```python
from build123d import *

# Parameters (mm, degrees)
F1_DEPTH = 47.752
F2_W     = 87.7630114555
F2_H     = 47.5155450404
F3_DEPTH = 32.004


with BuildPart() as f1:
    # F0 (on Right) → F1 (new body, symmetric)
    with BuildSketch(Plane.YZ):
        Polygon((-31.8501219153, 36.2352915108), (-27.2341612726, -24.6953871101), (43.6497934896, -30.3766369124), (46.6212034225, -24.6953871101), (-19.860636737, -19.3669606344), (-24.1173089374, 36.8211106937), align=None)
    extrude(amount=F1_DEPTH, both=True)

    # F2 (on face) → F3 (cut)
    with BuildSketch(Plane(origin=(0, -21.2061243549, -1.6065246214), x_dir=(-1, 0, 0), z_dir=(0, 0.9971426879, 0.075541115))):
        with Locations((0.0438690186, 10.5752218515)):
            Rectangle(F2_W, F2_H)
    extrude(amount=-F3_DEPTH, mode=Mode.SUBTRACT)


solid = f1.part
```
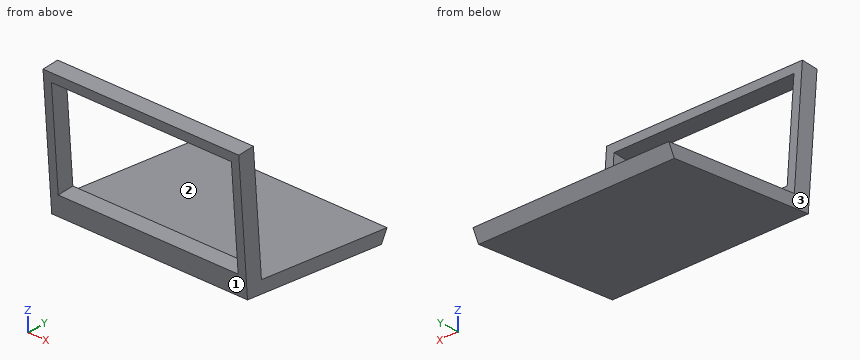
Work out the finished part from the listing and answer in its coordinate system (mm). Face numbers are marked on the shaded views. Round coordinates to 2 decimals unless told otherwise and drop trailing zeros. Order: outer loops, then holes, each group sorted by start corner. A loop starts at its lowest first (then second) coordinate and runs counter-clockwise, first axis right, second up.
Q1. The mould has two halves that part along Z. Classify the marked faces 1, 2 and 3: pulls with the +Z half, pulls with the -Z half, needs draft (parallel to the pull), parting line crosses it, or undercut.
Solution:
face 1: pulls with the -Z half
face 2: pulls with the +Z half
face 3: needs draft
Q2. A cutting plane is placed at A-A, the plane x = -36.5. Determine the outline of the cut face in (y, z), then the cut area to 3 significant figures.
Solution:
outline: (-31.85, 36.24) - (-31.53, 32.04) - (-23.8, 32.63) - (-24.12, 36.82) - close; (-27.94, -15.34) - (-27.23, -24.7) - (43.65, -30.38) - (46.62, -24.7) - (-19.86, -19.37) - (-20.21, -14.75) - close
area: 494 mm2
Q3. A cutting plane is placed at B-B, the plane z = 2. Determine the outline of the cut face in (x, y).
Solution:
outline: (-47.75, -29.26) - (-43.93, -29.26) - (-43.93, -21.48) - (-47.75, -21.48) - close; (43.84, -29.26) - (47.75, -29.26) - (47.75, -21.48) - (43.84, -21.48) - close
Q4. A cutting plane is placed at C-C, the plane y = 7.5. Determine the outline of the cut face in (x, z), then the cut area to 3 significant figures.
Solution:
outline: (-47.75, -27.48) - (47.75, -27.48) - (47.75, -21.56) - (-47.75, -21.56) - close
area: 565 mm2
Q5. Given pin 1 Ø1 at (x, y) = (22, 23.5) entering from +Z; pin 2 Ø1.5 at (x, y) = (-6, -16.5) entering from +Z; pin 3 Ø1.5 at (x, y) = (-19.5, -9) entering from -Z, each flat-ended and moving along its own axis, determine where each tip first touches the part or whether it passes through.
Solution:
pin 1: stops at z = -22.8
pin 2: stops at z = -19.58
pin 3: stops at z = -26.22
Q6. Find the intervals of material crossed by line 1 along X through (y, z) = (-25, 31); line 2 along Z through (x, y) = (-0.5, -24.5); line 3 along Z through (x, y) = (41, 5), in increasing order.
Solution:
line 1: x = -47.75 to -43.93, 43.84 to 47.75
line 2: z = -24.91 to -15.08, 32.58 to 36.79
line 3: z = -27.28 to -21.36
